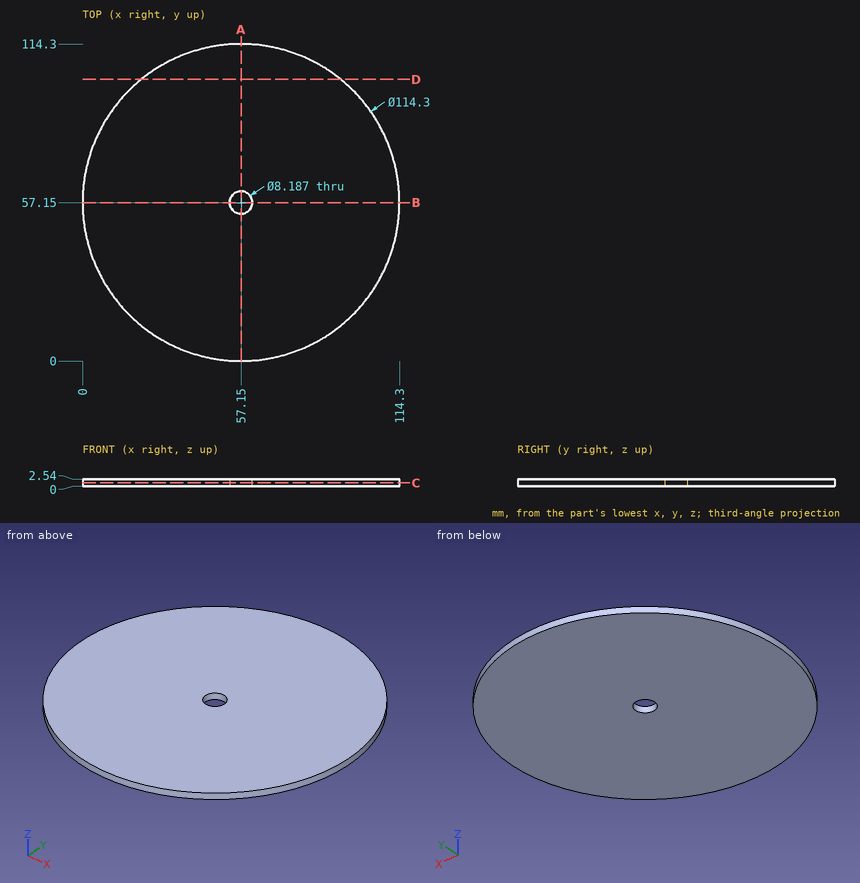
Could you check a few things on this drawing? It's one solid part, dimensions in mm from its lowest x, y, z. Coordinates: 2 decimals unless noted, no trailing zeros. Write each loop counter-clockwise with the first axis right and the second up, starting at its lowest first coordinate (ties: lowest second). Pieces come first, ordered by that corner, then holes. Notation, with made-up numbers: (77, 21) - (83, 21) arc R14 cw to (83, 25) - close; hole circle Ø6 at (82, -6.5). An arc over 180 degrees is marked (long way). Use one line per item in the form item = value.
1) Suppose I cut it at A-A, the plane x = 57.15. Write out the boundary of the cut face in (y, z).
Solved:
outline = (0, 0) - (53.06, 0) - (53.06, 2.54) - (0, 2.54) - close; (61.24, 0) - (114.3, 0) - (114.3, 2.54) - (61.24, 2.54) - close
2) Suppose I cut it at C-C, the plane z = 1.1. Write out the boundary of the cut face in (x, y).
Solved:
outline = circle Ø114.3 at (57.15, 57.15); hole circle Ø8.19 at (57.15, 57.15)
3) I'm going to push flat-ended pins straight in: P1, Ø1.5, axis at x = 85, z = 0.5, coming from the -Y side; P2, Ø7.5, axis at x = 57.15, y = 57.15, coming from the +Z side; P3, Ø1.5, axis at x = 95, z = 1.5, coming from the -Y side; P4, Ø1, axis at y = 72, z = 1.5, coming from the +X side. Where does each tip first touch, or does it pass through?
Solved:
P1 = 6.83
P2 = through
P3 = 13.68
P4 = 112.47
4) Suppose I cut it at D-D, the plane y = 101.5. Write out the boundary of the cut face in (x, z) (1 decimal), plus the area to 3 significant figures.
Solved:
outline = (21.1, 0) - (93.2, 0) - (93.2, 2.5) - (21.1, 2.5) - close
area = 183 mm2
5) I need wall thicknesses on line 1 (Y direction, x = 57.15, z = 1.55); line 2 (X direction, y = 46.5, z = 2.2); line 3 (X direction, y = 10, z = 1.9) (1 decimal). Which ranges of each line are inside material? Lowest first, please.
Solved:
line_1 = 0 to 53.06, 61.24 to 114.3
line_2 = 1 to 113.3
line_3 = 24.9 to 89.4
